Read the model definition and answer for the solid it produces. Units are mm, in the model's axes. A direction names the side the tool comes from. Give positions to 0.01 mm unless a question says otherwise; leave off trailing zeros. Order: outer loops, then holes, each group sorted by start corner. A loop starts at its lowest first (then second) coordinate and runs counter-clockwise, first axis right, second up.
```python
from build123d import *

# Parameters (mm, degrees)
SKETCH1_R           = 9.525
BOSS_EXTRUDE1_DEPTH = 3.556
FILLET1_R           = 19.05
CHAMFER2_SIZE       = 0.762


with BuildPart() as part:
    # Sketch1 → Boss-Extrude1 (new body, symmetric)
    with BuildSketch(Plane.XY):
        with BuildLine():
            Line((-31.75, 7.366), (-31.75, -7.366))
            Line((-31.75, -7.366), (-10.345629222, -7.366))
            ThreePointArc((-10.345629222, -7.366), (12.7, 0), (-10.345629222, 7.366))
            Line((-10.345629222, 7.366), (-31.75, 7.366))
        make_face()
        Circle(SKETCH1_R, mode=Mode.SUBTRACT)
    extrude(amount=BOSS_EXTRUDE1_DEPTH, both=True)

    # Fillet1
    fillet1_edges = [part.edges().sort_by_distance(p)[0] for p in [
        (-10.345629222, 7.366, 0),
        (-10.345629222, -7.366, 0),
    ]]
    fillet(fillet1_edges, radius=FILLET1_R)

    # Chamfer2
    chamfer2_edges = [part.edges().sort_by_distance(p)[0] for p in [
        (-24.682063131, -7.366, 3.556),
        (-24.682063131, 7.366, -3.556),
        (-24.682063131, 7.366, 3.556),
        (12.7, 0, -3.556),
        (12.7, 0, 3.556),
        (-12.092911722, 8.183647162, -3.556),
        (-12.092911722, 8.183647162, 3.556),
        (-12.092911722, -8.183647162, -3.556),
        (-12.092911722, -8.183647162, 3.556),
        (-24.682063131, -7.366, -3.556),
        (-31.75, 0, -3.556),
        (-31.75, -7.366, 0),
        (-31.75, 7.366, 0),
        (-31.75, 0, 3.556),
    ]]
    chamfer(chamfer2_edges, length=CHAMFER2_SIZE)

    # Sketch2 → Cut-Revolve1 (revolve, cut)
    with BuildSketch(Plane(origin=(0, 0, 0), x_dir=(1, 0, 0), z_dir=(0, 1, 0))):
        with BuildLine():
            Line((10.646210245, 3.556), (10.302407684, 3.212197439))
            ThreePointArc((10.302407684, 3.212197439), (10.212605122, 3.175), (10.122802561, 3.212197439))
            Line((10.122802561, 3.212197439), (9.779, 3.556))
            Line((9.779, 3.556), (10.646210245, 3.556))
        make_face()
    cut_revolve1 = revolve(axis=Axis((0, 0, -14.192615474), (0, 0, 1)), mode=Mode.SUBTRACT)

    # Mirror1: Cut-Revolve1 across plane
    add(cut_revolve1.mirror(Plane.XY), mode=Mode.SUBTRACT)


solid = part.part
```
1) The part is cut by section A-A on y = 0. Determine the outline of the cut face in (x, z) (3 decimals).
Final values:
outline: (-31.75, -2.794) - (-30.988, -3.556) - (-10.646, -3.556) - (-10.302, -3.212) arc R0.127 cw to (-10.123, -3.212) - (-9.779, -3.556) - (-9.525, -3.556) - (-9.525, 3.556) - (-9.779, 3.556) - (-10.123, 3.212) arc R0.127 cw to (-10.302, 3.212) - (-10.646, 3.556) - (-30.988, 3.556) - (-31.75, 2.794) - close; (9.525, -3.556) - (9.779, -3.556) - (10.123, -3.212) arc R0.127 cw to (10.302, -3.212) - (10.646, -3.556) - (11.938, -3.556) - (12.7, -2.794) - (12.7, 2.794) - (11.938, 3.556) - (10.646, 3.556) - (10.302, 3.212) arc R0.127 cw to (10.123, 3.212) - (9.779, 3.556) - (9.525, 3.556) - close
2) The part is cut by section D-D on x = -21. Determine the outline of the cut face in (y, z).
Final values:
outline: (-7.37, -2.79) - (-6.6, -3.56) - (6.6, -3.56) - (7.37, -2.79) - (7.37, 2.79) - (6.6, 3.56) - (-6.6, 3.56) - (-7.37, 2.79) - close
3) Consider L1, parallel to Y at x = 0, z = 1.75 (3 decimals); L2, parallel to X at y = 0.5, z = 3.25; L3, parallel to Y at x = 5.5, z = -3. Determine where each line is inside the solid, lowest interval first.
Final values:
L1: y = -12.7 to -9.525, 9.525 to 12.7
L2: x = -31.29 to -10.33, -10.07 to -9.51, 9.51 to 10.07, 10.33 to 12.23
L3: y = -11.22 to -7.78, 7.78 to 11.22
4) Given pin 1 (11.5 mm diameter, centred on x = 0, y = 0, fed in from -Z); pin 2 (1.5 mm diameter, centred on y = 5, z = 1.5, fed in from +X); pin 3 (2 mm diameter, centred on y = -3.5, z = 1.5, fed in from +X); pin 4 (1.7 mm diameter, centred on x = -25.5, z = 0, fed in from +Y), each flat-ended and moving along its own axis, determine where each tip first touches the part or whether it passes through.
Final values:
pin 1: passes through
pin 2: stops at x = 11.97
pin 3: stops at x = 12.45
pin 4: stops at y = 7.37
5) The part is cut by section B-B on x = 0. Determine the outline of the cut face in (y, z) (3 decimals), and give its area (3 significant figures).
Final values:
outline: (-12.7, -2.794) - (-11.938, -3.556) - (-10.646, -3.556) - (-10.302, -3.212) arc R0.127 cw to (-10.123, -3.212) - (-9.779, -3.556) - (-9.525, -3.556) - (-9.525, 3.556) - (-9.779, 3.556) - (-10.123, 3.212) arc R0.127 cw to (-10.302, 3.212) - (-10.646, 3.556) - (-11.938, 3.556) - (-12.7, 2.794) - close; (9.525, -3.556) - (9.779, -3.556) - (10.123, -3.212) arc R0.127 cw to (10.302, -3.212) - (10.646, -3.556) - (11.938, -3.556) - (12.7, -2.794) - (12.7, 2.794) - (11.938, 3.556) - (10.646, 3.556) - (10.302, 3.212) arc R0.127 cw to (10.123, 3.212) - (9.779, 3.556) - (9.525, 3.556) - close
area: 43.3 mm2
6) For a pull along X with two mould halves and no side action, classify faces 1 (the face through (12.694, -0.384, 0.039)), 2 (the face through (-7.559, -5.796, -0.05)), 3 (the face through (-12.018, -8.207, 0.039)), 4 (the face through (-24, 7.366, 0)) as released by +X, released by -X, zero draft, split by the parting line, or undercut.
Final values:
face 1: split by the parting line
face 2: undercut
face 3: released by -X
face 4: zero draft
7) The part is cut by section C-C on z = -2.25. Determine the outline of the cut face in (x, y) (3 decimals).
Final values:
outline: (-31.75, -6.604) - (-30.988, -7.366) - (-17.614, -7.366) arc R19.05 cw to (-7.046, -10.566) arc R12.7 ccw (long way) to (-7.046, 10.566) arc R19.05 cw to (-17.614, 7.366) - (-30.988, 7.366) - (-31.75, 6.604) - close; hole circle Ø19.05 at (0, 0)
8) A tool of negligible diameter and unlimited length cuts with its end or side. For faces 5 (the face through (-24, -7.366, 0)), 6 (the face through (-15, 0, 3.556)), from which of +Z, -Z, +X, -X, +Y, -Y can it reach the whole face along a straight path? Write none if from no direction.
Final values:
face 5: +Z, -Z, -X, -Y
face 6: +Z, +X, -X, +Y, -Y
